Design review of the part built by this model. Coordinates are the model's own, in mm. Face numbers are marked on the shaded views. A direction names the side the tool comes from. Coordinates: 2 decimals unless noted, no trailing zeros. Loops run counter-clockwise (first coordinate to the right, second up) from the corner with the lowest first, then second, coordinate; pieces in that order, holes last.
Q1. Add section A-A on x = 0. Give the boundary of the cut face in (y, z).
Q2. For P1, Ø6, axis at x = 7.5, y = 4.5, coming from the +Z side; P2, Ø5, axis at x = -37.5, y = 5.5, coming from the -Z side; P3, Ø2, axis at x = 14.5, y = 4, coming from the -Z side, all flat-tipped, find the tip position at first contact; note any pin that passes through.
Q3. Add section C-C on x = 37. Give the boundary of the cut face in (y, z), and give its area (3 significant figures).
Q4. Machinability: for the marked faces 4 and 5, which of the approach directions +Z, -Z, +X, -X, +Y, -Y give a long, thin tool a straight path to every point of the face, cutting with its end or side? Answer none if there is none.
Q5. Add section D-D on y = 10. Give the number of separate pieces and of enclosed holes in the cut face, and give its area (3 significant figures).
Q6. Draft analysis for pull direction X (two halves, no side actions). For the marked faces 1, 2 and 3, state which applies: released by +X, released by -X, zero draft, split by the parting line, or undercut.
Q7. Add section B-B on z = 0. Give the boundary of the cut face in (x, y), and give its area (3 significant figures).
Q8. Wall thickness on probe 1 along X at (y, z) = (10.25, 11); probe 2 along X at (y, z) = (2.5, 10.5); probe 3 along Z at (x, y) = (-18.5, 13.5): over which ranges is each line inside the solid? List them lowest first.
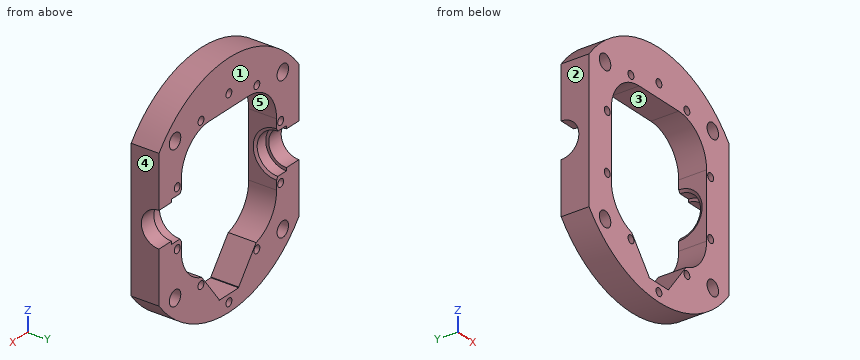
```python
from build123d import *
from OCP.BRepFilletAPI import BRepFilletAPI_MakeChamfer

# Parameters (mm, degrees)
SKETCH2_R               = 62.5
SKETCH2_W               = 68.2
SKETCH2_H               = 75
BOSS_EXTRUDE1_DEPTH     = 15
SKETCH7_W               = 7
SKETCH7_H               = 11.1
CUT_EXTRUDE1_DEPTH      = 122.918866465
CUT_EXTRUDE1_DEPTH_BACK = 122.918866465
SKETCH8_R               = 9.5
FILLET1_R               = 20
SKETCH9_R               = 2.1
CUT_EXTRUDE2_DEPTH      = 90.652105542
CHAMFER1_SIZE           = 1.5
CHAMFER1_SIZE2          = 0.866025404
SKETCH10_R              = 4.1
CUT_EXTRUDE3_DEPTH      = 90.652105542
CUT_EXTRUDE4_DEPTH      = 90.652105542
SKETCH12_W              = 14
SKETCH12_H              = 16
CUT_EXTRUDE5_DEPTH      = 90.652105542
CHAMFER2_DEPTH          = 15
CUT_EXTRUDE6_DEPTH      = 90.652105542


with BuildPart() as part:
    # Sketch2 → Boss-Extrude1 (new body)
    with BuildSketch(Plane(origin=(0, 0, 0), x_dir=(1, 0, 0), z_dir=(0, 1, 0))):
        with Locations(Location((0, 0, 0), (0, 0, 270))):
            Circle(SKETCH2_R)
        Rectangle(SKETCH2_W, SKETCH2_H, mode=Mode.SUBTRACT)
    extrude(amount=BOSS_EXTRUDE1_DEPTH)

    # Sketch7 → Cut-Revolve2 (revolve, cut)
    with BuildSketch(Plane(origin=(0, 15, 0), x_dir=(1, 0, 0), z_dir=(0, 1, 0))):
        with Locations((-37.6, 5.55)):
            Rectangle(SKETCH7_W, SKETCH7_H)
        with Locations((37.6, 5.55)):
            Rectangle(SKETCH7_W, SKETCH7_H)
    revolve(axis=Axis((62.5, 15, 0), (-1, 0, 0)), mode=Mode.SUBTRACT)

    # Sketch8 → Cut-Extrude1 (cut, two sides: drawn at the far end of the back side and taken through both)
    with BuildSketch(Plane.ZY.offset(-41.1).offset(-CUT_EXTRUDE1_DEPTH_BACK)):
        with Locations((0, 15)):
            Circle(SKETCH8_R)
    extrude(amount=CUT_EXTRUDE1_DEPTH + CUT_EXTRUDE1_DEPTH_BACK, mode=Mode.SUBTRACT)

    # Fillet1
    fillet1_edges = [part.edges().sort_by_distance(p)[0] for p in [
        (-34.1, 7.5, -37.5),
        (-34.1, 7.5, 37.5),
        (34.1, 7.5, 37.5),
        (34.1, 7.5, -37.5),
    ]]
    fillet(fillet1_edges, radius=FILLET1_R)

    # Sketch9 → Cut-Extrude2 (cut, through all)
    with BuildSketch(Plane(origin=(0, 15, 0), x_dir=(1, 0, 0), z_dir=(0, 1, 0))):
        with Locations(Location((-37, 15.198684154, 0), (0, 0, 270))):
            Circle(SKETCH9_R)
        with Locations(Location((37, 15.198684154, 0), (0, 0, 270))):
            Circle(SKETCH9_R)
        with Locations(Location((37, -15.198684154, 0), (0, 0, 270))):
            Circle(SKETCH9_R)
        with Locations(Location((-37, -15.198684154, 0), (0, 0, 270))):
            Circle(SKETCH9_R)
        with Locations(Location((-20, 40.311288741, 0), (0, 0, 270))):
            Circle(SKETCH9_R)
        with Locations(Location((20, 40.311288741, 0), (0, 0, 270))):
            Circle(SKETCH9_R)
        with Locations(Location((20, -40.311288741, 0), (0, 0, 270))):
            Circle(SKETCH9_R)
        with Locations(Location((-20, -40.311288741, 0), (0, 0, 270))):
            Circle(SKETCH9_R)
        with Locations(Location((0, -45, 0), (0, 0, 270))):
            Circle(SKETCH9_R)
        with Locations(Location((0, 57.5, 0), (0, 0, 270))):
            Circle(SKETCH9_R)
    extrude(amount=-CUT_EXTRUDE2_DEPTH, mode=Mode.SUBTRACT)

    # Chamfer1: one chamfer whose edges measure the first distance from different faces: ONE call of the kernel's chamfer builder (chamfer() names one face for all edges)
    chamfer1_edges_1 = [part.edges().sort_by_distance(p)[0] for p in [
        (-34.1, 3.9, 0),
    ]]
    chamfer1_side_1 = [part.faces().sort_by_distance(p)[0] for p in [
        (-34.1, 0.380788655, 0),
    ]]
    chamfer1_edges_2 = [part.edges().sort_by_distance(p)[0] for p in [
        (34.1, 3.9, 0),
    ]]
    chamfer1_side_2 = [part.faces().sort_by_distance(p)[0] for p in [
        (34.1, 0.380788655, 0),
    ]]
    chamfer1 = BRepFilletAPI_MakeChamfer(part.part.solid().wrapped)
    for e in chamfer1_edges_1:
        chamfer1.Add(CHAMFER1_SIZE, CHAMFER1_SIZE2, e.wrapped, chamfer1_side_1[0].wrapped)  # the first distance lies on this face
    for e in chamfer1_edges_2:
        chamfer1.Add(CHAMFER1_SIZE, CHAMFER1_SIZE2, e.wrapped, chamfer1_side_2[0].wrapped)  # the first distance lies on this face
    add(Compound.cast(chamfer1.Shape()), mode=Mode.REPLACE)

    # Sketch10 → Cut-Extrude3 (cut, through all)
    with BuildSketch(Plane.XZ):
        with Locations(Location((38.537319575, -38.537319575, 0), (0, 0, 270))):
            Circle(SKETCH10_R)
        with Locations(Location((-38.537319575, -38.537319575, 0), (0, 0, 270))):
            Circle(SKETCH10_R)
        with Locations(Location((-38.537319575, 38.537319575, 0), (0, 0, 270))):
            Circle(SKETCH10_R)
        with Locations(Location((38.537319575, 38.537319575, 0), (0, 0, 270))):
            Circle(SKETCH10_R)
    extrude(amount=-CUT_EXTRUDE3_DEPTH, mode=Mode.SUBTRACT)

    # Sketch11 → Cut-Extrude4 (cut, through all)
    with BuildSketch(Plane.XZ):
        with BuildLine():
            Line((50, -37.5), (50, 37.5))
            ThreePointArc((50, 37.5), (62.5, 0), (50, -37.5))
        make_face()
    extrude(amount=-CUT_EXTRUDE4_DEPTH, mode=Mode.SUBTRACT)

    # Sketch12 → Cut-Extrude5 (cut, through all)
    with BuildSketch(Plane(origin=(0, 15, 0), x_dir=(1, 0, 0), z_dir=(0, 1, 0))):
        with Locations((0, 45.5)):
            Rectangle(SKETCH12_W, SKETCH12_H)
    extrude(amount=-CUT_EXTRUDE5_DEPTH, mode=Mode.SUBTRACT)

    # Chamfer2: read off the stored shape, not the designer's step
    # Chamfer2 outline → Chamfer2 (cut)
    with BuildSketch(Plane(origin=(0, 0, 0), x_dir=(1, 0, 0), z_dir=(0, 1, 0))):
        with BuildLine():
            ThreePointArc((14.1, 37.5), (16.800403682, 37.316856965), (19.451351351, 36.770781996))
            Line((19.451351351, 36.770781996), (7, 53.150946691))
            Line((7, 53.150946691), (7, 37.5))
            Line((7, 37.5), (14.1, 37.5))
        make_face()
        with BuildLine():
            Line((-7, 37.5), (-7, 53.150946691))
            Line((-7, 53.150946691), (-19.451351351, 36.770781996))
            ThreePointArc((-19.451351351, 36.770781996), (-16.800403682, 37.316856965), (-14.1, 37.5))
            Line((-14.1, 37.5), (-7, 37.5))
        make_face()
    extrude(amount=CHAMFER2_DEPTH, mode=Mode.SUBTRACT)

    # Sketch13 → Cut-Extrude6 (cut, through all)
    with BuildSketch(Plane.XZ):
        with BuildLine():
            Line((-50, -37.5), (-50, 37.5))
            ThreePointArc((-50, 37.5), (-62.5, 0), (-50, -37.5))
        make_face()
    extrude(amount=-CUT_EXTRUDE6_DEPTH, mode=Mode.SUBTRACT)


solid = part.part
```
Entries:
1. outline: (0, -62.5) - (15, -62.5) - (15, -59.6) - (0, -59.6) - close; (0, -55.4) - (15, -55.4) - (15, -53.5) - (0, -53.5) - close; (0, 37.5) - (15, 37.5) - (15, 42.9) - (0, 42.9) - close; (0, 47.1) - (15, 47.1) - (15, 62.5) - (0, 62.5) - close
2. P1: stops at z = 62.34
2. P2: stops at z = -51.78
2. P3: stops at z = -61.02
3. outline: (0, -50.37) - (15, -50.37) - (15, -42.34) - (0, -42.34) - close; (0, -34.74) - (15, -34.74) - (15, -17.3) - (0, -17.3) - close; (0, -13.1) - (15, -13.1) - (15, -11.1) arc R11.1 cw to (15, 11.1) - (15, 13.1) - (0, 13.1) - close; (0, 17.3) - (15, 17.3) - (15, 34.74) - (0, 34.74) - close; (0, 42.34) - (15, 42.34) - (15, 50.37) - (0, 50.37) - close
3. area: 964 mm2
4. face 4: +Z, -Z, +X, +Y, -Y
4. face 5: +Y, -Y
5. separate pieces: 2
5. enclosed holes: 14
5. area: 4,890 mm2
6. face 1: zero draft
6. face 2: released by -X
6. face 3: undercut
7. outline: (-50, 0) - (-34.1, 0) - (-34.1, 2.4) - (-34.97, 3.9) - (-41.1, 3.9) - (-41.1, 5.5) - (-50, 5.5) - close; (34.1, 0) - (50, 0) - (50, 5.5) - (41.1, 5.5) - (41.1, 3.9) - (34.97, 3.9) - (34.1, 2.4) - close
7. area: 151 mm2
8. probe 1: x = -50 to -34.46, 34.46 to 50
8. probe 2: x = -50 to -34.1, 34.1 to 50
8. probe 3: z = -59.7 to -41.78, -38.84 to -38.02, 37.01 to 38.84, 41.78 to 59.7
